Can you work these out from the drawing? Everything is in mm from the part's minimum corner. A direction names the side the tool comes from. Round coordinates to 2 decimals unless told otherwise and drop trailing zeros. Write each loop counter-clockwise with the first axis right and the second up, starting at its lowest first coordinate (ties: lowest second). Pieces come first, ordered by that corner, then holes. Notation, with made-up numbers: (65, -6.5) -> (85, -6.5) arc R19 cw to (85, 14.5) -> close; hole circle Ø11 at (-29, 39). An arc over 180 degrees is marked (long way). Write item = value, one per line. Start each with the question number.
1) I'm going to push flat-ended pins straight in: pin 1 (11.5 mm diameter, centred on x = 40, z = 40, fed in from -Y); pin 2 (6 mm diameter, centred on y = 5.5, z = 67.5, fed in from +X); pin 3 (1.5 mm diameter, centred on x = 23, y = 8.5, fed in from +Z); pin 4 (1.5 mm diameter, centred on y = 8, z = 12, fed in from -X). Where does each tip first touch, or does it pass through?
2) Imagine slicing it at D-D, the plane y = 6.75. Please give me the cut outline in (x, z), then the cut area to 3 significant figures.
3) Imagine slicing it at C-C, the plane y = 12.5. Please give me the cut outline in (x, z) (1 decimal).
4) If I drill on line 1 (X direction, y = 8.25, z = 40); line 2 (Y direction, x = 67, z = 38); line 3 (Z direction, x = 56, y = 11.25), over which ranges is the centre line in solid material (lowest first)?
5) Imagine slicing it at B-B, the plane x = 40. Please give me the cut outline in (y, z), then the cut area to 3 significant figures.
6) Imagine slicing it at A-A, the plane z = 40. Please give me the cut outline in (x, y).
7) Thinking about a two-plate mould opening in Z: for the marked faces 1, 2 and 3, which applies, +Z half, -Z half, draft (parallel to the pull), parting line (faces both ways), or undercut?
8) For the marked faces 4 and 5, which set-ups out of +Z, -Z, +X, -X, +Y, -Y let a thin tool reach every point of the face, with its end or its side?
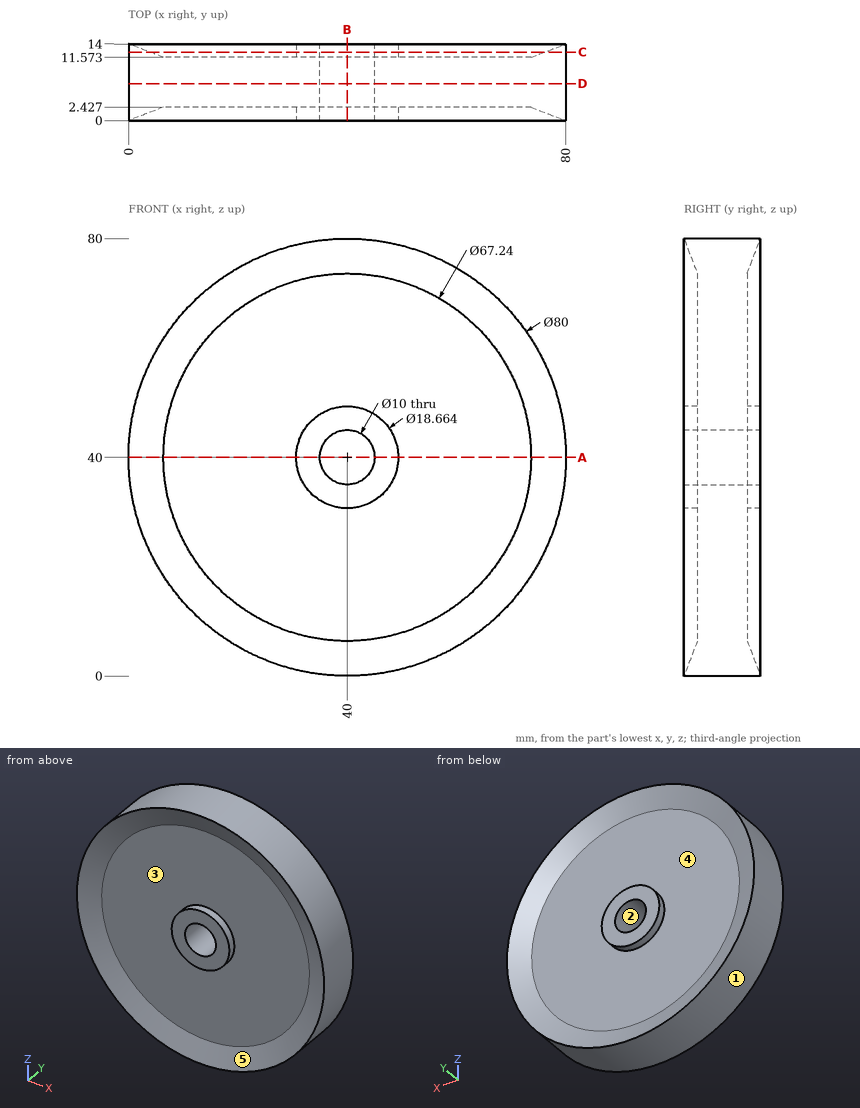
Reported:
q1.pin_1 = 0
q1.pin_2 = 71.62
q1.pin_3 = 76.55
q1.pin_4 = 10.72
q2.outline = circle Ø80 at (40, 40); hole circle Ø10 at (40, 40)
q2.area = 4,950 mm²
q3.outline = circle Ø80 at (40, 40); circle Ø18.7 at (40, 40); hole circle Ø72.1 at (40, 40); hole circle Ø10 at (40, 40)
q4.line_1 = 0 to 35, 45 to 80
q4.line_2 = 2.43 to 11.57
q4.line_3 = 3.34 to 76.66
q5.outline = (0, 0) -> (14, 0) -> (11.57, 6.38) -> (11.57, 30.67) -> (14, 30.67) -> (14, 35) -> (0, 35) -> (0, 30.67) -> (2.43, 30.67) -> (2.43, 6.38) -> close; (0, 45) -> (14, 45) -> (14, 49.33) -> (11.57, 49.33) -> (11.57, 73.62) -> (14, 80) -> (0, 80) -> (2.43, 73.62) -> (2.43, 49.33) -> (0, 49.33) -> close
q5.area = 713 mm²
q6.outline = (0, 0) -> (6.38, 2.43) -> (30.67, 2.43) -> (30.67, 0) -> (35, 0) -> (35, 14) -> (30.67, 14) -> (30.67, 11.57) -> (6.38, 11.57) -> (0, 14) -> close; (45, 0) -> (49.33, 0) -> (49.33, 2.43) -> (73.62, 2.43) -> (80, 0) -> (80, 14) -> (73.62, 11.57) -> (49.33, 11.57) -> (49.33, 14) -> (45, 14) -> close
q7.face_1 = parting line
q7.face_2 = undercut
q7.face_3 = undercut
q8.face_4 = +Y
q8.face_5 = -Y
